Source: CAD feature listing. Evaluate the final solid. Frame: model axes, mm. Face numbers are marked on the shaded views. A direction names the side the tool comes from. Give positions to 0.01 mm unless a question says otherwise; leave off trailing zeros. Order: outer loops, then holes, each group sorted by start corner. A loop starts at its lowest first (then second) coordinate and runs counter-clockwise, first axis right, second up.
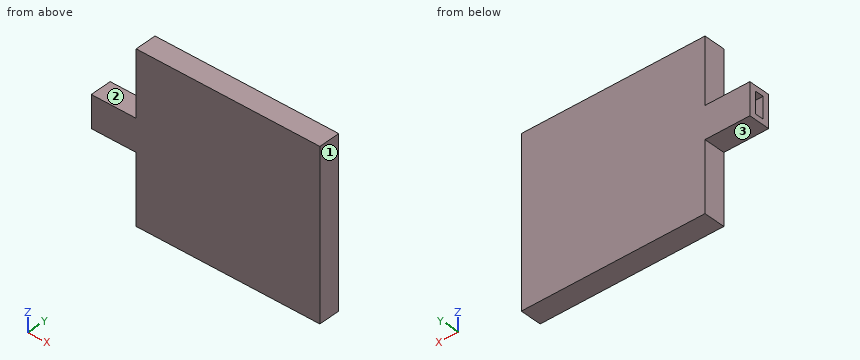
from build123d import *

# Parameters (mm, degrees)
BOSS_EXTRUDE1_DEPTH = 5
SKETCH3_W           = 5
SKETCH3_H           = 2
CUT_EXTRUDE1_DEPTH  = 14


with BuildPart() as part:
    # Sketch1 → Boss-Extrude1 (new body)
    with BuildSketch(Plane(origin=(0, 0, 0), x_dir=(1, 0, 0), z_dir=(0, 1, 0))):
        Polygon((0, 22.75), (-10.5, 22.75), (-10.5, 15.25), (0, 15.25), (0, 0), (43, 0), (43, 39), (0, 39), align=None)
    extrude(amount=BOSS_EXTRUDE1_DEPTH)

    # Sketch3 → Cut-Extrude1 (cut)
    with BuildSketch(Plane.ZY.offset(10.5)):
        with Locations((-19, 2.5)):
            Rectangle(SKETCH3_W, SKETCH3_H)
    extrude(amount=-CUT_EXTRUDE1_DEPTH, mode=Mode.SUBTRACT)


solid = part.part
1) Reachability of the marked faces 1, 2 and 3 from +Z, -Z, +X, -X, +Y, -Y: full face, straight path, thin tool, end or side. Return the list, or none.
Checks:
face 1: +Z, -Z, +X, +Y, -Y
face 2: +Z, -X, +Y, -Y
face 3: -Z, -X, +Y, -Y
2) Section query A-A on z = -20. Output: boundary loops of the cut face in (x, y).
Checks:
outline: (-10.5, 0) - (43, 0) - (43, 5) - (-10.5, 5) - (-10.5, 3.5) - (3.5, 3.5) - (3.5, 1.5) - (-10.5, 1.5) - close
3) Section query B-B on x = -6. Output: boundary loops of the cut face in (y, z).
Checks:
outline: (0, -22.75) - (5, -22.75) - (5, -15.25) - (0, -15.25) - close; hole (1.5, -21.5) - (3.5, -21.5) - (3.5, -16.5) - (1.5, -16.5) - close
4) Section query C-C on y = 2.75. Output: boundary loops of the cut face in (x, z).
Checks:
outline: (-10.5, -22.75) - (0, -22.75) - (0, -39) - (43, -39) - (43, 0) - (0, 0) - (0, -15.25) - (-10.5, -15.25) - (-10.5, -16.5) - (3.5, -16.5) - (3.5, -21.5) - (-10.5, -21.5) - close
5) First-contact query: pin 1 Ø1.5 at (x, y) = (-4, 3) entering from +Z; pin 2 Ø1.5 at (y, z) = (3, -10.5) entering from -X; pin 3 Ø1 at (y, z) = (2.5, -20) entering from -X. Flat tips, straight axial feed; report the tip coordinate or a pass-through.
Checks:
pin 1: stops at z = -15.25
pin 2: stops at x = 0
pin 3: stops at x = 3.5
6) Section query D-D on z = -33.5. Output: boundary loops of the cut face in (x, y), and give its area (3 significant figures).
Checks:
outline: (0, 0) - (43, 0) - (43, 5) - (0, 5) - close
area: 215 mm2
7) Ray query, L1, parallel to X at y = 0.7, z = -30; L2, parallel to X at y = 1.7, z = -19.5; L3, parallel to Z at x = -8, y = 1.4. Return the intervals inside material, ascending.
Checks:
L1: x = 0 to 43
L2: x = 3.5 to 43
L3: z = -22.75 to -15.25
